from build123d import *

# Parameters (mm, degrees)
F0_W         = 76.2
F0_H         = 101.6
F1_DEPTH     = 38.1
F2_W         = 69.85
F2_H         = 95.25
F3_DEPTH     = 34.925
F4_W         = 72.39
F4_H         = 97.79
F4_W_2       = 69.85
F4_H_2       = 95.25
F5_DEPTH     = 3.175
F6_W         = 76.2
F6_H         = 101.6
F6_W_2       = 73.66
F6_H_2       = 99.06
F7_DEPTH     = 3.175
F8_T1_DEPTH  = 110.49
F8_T3_DEPTH  = 85.09
F8_T5_DEPTH  = 99.06
F8_T7_DEPTH  = 73.66
F8_T13_DEPTH = 105.41
F8_T19_DEPTH = 80.01
F8_T28_DEPTH = 105.41
F8_T34_DEPTH = 80.01
F8_T43_DEPTH = 80.01
F8_T49_DEPTH = 105.41
F8_T58_DEPTH = 105.41
F8_T64_DEPTH = 80.01


# Not quite as in the source:
# - a fillet or chamfer that OpenCascade refuses, or shapes differently, is made with other operations: its cross-section is extruded or revolved along the edge and cut away or added


with BuildPart() as f1:
    # F0 (on Top) → F1 (new body)
    with BuildSketch(Plane.XY):
        Rectangle(F0_W, F0_H)
    extrude(amount=F1_DEPTH)

    # F2 (on face) → F3 (cut)
    with BuildSketch(Plane.XY.offset(38.1)):
        Rectangle(F2_W, F2_H)
    extrude(amount=-F3_DEPTH, mode=Mode.SUBTRACT)

    # F4 (on face) → F5 (join)
    with BuildSketch(Plane.XY.offset(38.1)):
        Rectangle(F4_W, F4_H)
        Rectangle(F4_W_2, F4_H_2, mode=Mode.SUBTRACT)
    extrude(amount=F5_DEPTH)

    # F6 (on face) → F7 (join)
    with BuildSketch(Plane(origin=(0, 0, 0), x_dir=(1, 0, 0), z_dir=(0, 0, -1))):
        Rectangle(F6_W, F6_H)
        Rectangle(F6_W_2, F6_H_2, mode=Mode.SUBTRACT)
    extrude(amount=F7_DEPTH)

    # F8: fillet of radius 2.54 on 8 edges, made by hand

    # F8_s2 → F8_t1 (cut)
    with BuildSketch(Plane.XZ.offset(-55.245)):
        with BuildLine():
            ThreePointArc((-33.655, 41.275), (-35.4510512242, 40.5310512242), (-36.195, 38.735))
            Line((-36.195, 38.735), (-36.195, 41.275))
            Line((-36.195, 41.275), (-33.655, 41.275))
        make_face()
        with BuildLine():
            ThreePointArc((36.195, 38.735), (35.4510512242, 40.5310512242), (33.655, 41.275))
            Line((33.655, 41.275), (36.195, 41.275))
            Line((36.195, 41.275), (36.195, 38.735))
        make_face()
    extrude(amount=F8_T1_DEPTH, mode=Mode.SUBTRACT)

    # F8_s4 → F8_t3 (cut)
    with BuildSketch(Plane.YZ.offset(-42.545)):
        with BuildLine():
            ThreePointArc((-46.355, 41.275), (-48.1510512242, 40.5310512242), (-48.895, 38.735))
            Line((-48.895, 38.735), (-48.895, 41.275))
            Line((-48.895, 41.275), (-46.355, 41.275))
        make_face()
        with BuildLine():
            ThreePointArc((46.355, 41.275), (48.1510512242, 40.5310512242), (48.895, 38.735))
            Line((48.895, 38.735), (48.895, 41.275))
            Line((48.895, 41.275), (46.355, 41.275))
        make_face()
    extrude(amount=F8_T3_DEPTH, mode=Mode.SUBTRACT)

    # F8_s6 → F8_t5 (cut)
    with BuildSketch(Plane.XZ.offset(-49.53)):
        with BuildLine():
            ThreePointArc((-39.37, -3.175), (-37.5739487758, -2.4310512242), (-36.83, -0.635))
            Line((-36.83, -0.635), (-36.83, -3.175))
            Line((-36.83, -3.175), (-39.37, -3.175))
        make_face()
        with BuildLine():
            ThreePointArc((39.37, -3.175), (37.5739487758, -2.4310512242), (36.83, -0.635))
            Line((36.83, -0.635), (36.83, -3.175))
            Line((36.83, -3.175), (39.37, -3.175))
        make_face()
    extrude(amount=F8_T5_DEPTH, mode=Mode.SUBTRACT)

    # F8_s8 → F8_t7 (cut)
    with BuildSketch(Plane.YZ.offset(-36.83)):
        with BuildLine():
            ThreePointArc((-52.07, -3.175), (-50.2739487758, -2.4310512242), (-49.53, -0.635))
            Line((-49.53, -0.635), (-49.53, -3.175))
            Line((-49.53, -3.175), (-52.07, -3.175))
        make_face()
        with BuildLine():
            ThreePointArc((52.07, -3.175), (50.2739487758, -2.4310512242), (49.53, -0.635))
            Line((49.53, -0.635), (49.53, -3.175))
            Line((49.53, -3.175), (52.07, -3.175))
        make_face()
    extrude(amount=F8_T7_DEPTH, mode=Mode.SUBTRACT)


with BuildPart() as f8_tool11:
    # F8_s12 → F8_t13 (new body)
    with BuildSketch(Plane.XZ.offset(-55.88)):
        with BuildLine():
            ThreePointArc((-39.37, -3.175), (-37.5739487758, -2.4310512242), (-36.83, -0.635))
            Line((-36.83, -0.635), (-36.83, -3.175))
            Line((-36.83, -3.175), (-39.37, -3.175))
        make_face()
    extrude(amount=F8_T13_DEPTH)

    split(bisect_by=Plane.XZ.offset(-49.53), keep=Keep.BOTTOM)

    split(bisect_by=Plane.YZ.offset(-38.1), keep=Keep.TOP)

    split(bisect_by=Plane.XZ.offset(-50.8), keep=Keep.TOP)


with BuildPart() as f8_tool17:
    # F8_s18 → F8_t19 (new body)
    with BuildSketch(Plane.YZ.offset(36.83)):
        with BuildLine():
            ThreePointArc((52.07, -3.175), (50.2739487758, -2.4310512242), (49.53, -0.635))
            Line((49.53, -0.635), (49.53, -3.175))
            Line((49.53, -3.175), (52.07, -3.175))
        make_face()
    extrude(amount=-F8_T19_DEPTH)

    split(bisect_by=Plane.YZ.offset(-36.83), keep=Keep.BOTTOM)

    split(bisect_by=Plane.YZ.offset(-38.1), keep=Keep.TOP)

    split(bisect_by=Plane.XZ.offset(-50.8), keep=Keep.TOP)


with BuildPart() as f8_tool11_1:
    add(f8_tool11.part)

    # F8_t23: intersect F8_tool17
    add(f8_tool17.part, mode=Mode.INTERSECT)


with BuildPart() as f1_1:
    add(f1.part)

    # F8_t9: cut F8_tool11
    add(f8_tool11_1.part, mode=Mode.SUBTRACT)


with BuildPart() as f8_tool26:
    # F8_s27 → F8_t28 (new body)
    with BuildSketch(Plane.XZ.offset(-49.53)):
        with BuildLine():
            ThreePointArc((-39.37, -3.175), (-37.5739487758, -2.4310512242), (-36.83, -0.635))
            Line((-36.83, -0.635), (-36.83, -3.175))
            Line((-36.83, -3.175), (-39.37, -3.175))
        make_face()
    extrude(amount=F8_T28_DEPTH)

    split(bisect_by=Plane.XZ.offset(49.53), keep=Keep.TOP)

    split(bisect_by=Plane.YZ.offset(-38.1), keep=Keep.TOP)

    split(bisect_by=Plane.XZ.offset(50.8), keep=Keep.BOTTOM)


with BuildPart() as f8_tool32:
    # F8_s33 → F8_t34 (new body)
    with BuildSketch(Plane.YZ.offset(-43.18)):
        with BuildLine():
            ThreePointArc((-52.07, -3.175), (-50.2739487758, -2.4310512242), (-49.53, -0.635))
            Line((-49.53, -0.635), (-49.53, -3.175))
            Line((-49.53, -3.175), (-52.07, -3.175))
        make_face()
    extrude(amount=F8_T34_DEPTH)

    split(bisect_by=Plane.YZ.offset(-36.83), keep=Keep.BOTTOM)

    split(bisect_by=Plane.YZ.offset(-38.1), keep=Keep.TOP)

    split(bisect_by=Plane.XZ.offset(50.8), keep=Keep.BOTTOM)


with BuildPart() as f8_tool26_1:
    add(f8_tool26.part)

    # F8_t38: intersect F8_tool32
    add(f8_tool32.part, mode=Mode.INTERSECT)


with BuildPart() as f1_2:
    add(f1_1.part)

    # F8_t24: cut F8_tool26
    add(f8_tool26_1.part, mode=Mode.SUBTRACT)


with BuildPart() as f8_tool41:
    # F8_s42 → F8_t43 (new body)
    with BuildSketch(Plane.YZ.offset(-36.83)):
        with BuildLine():
            ThreePointArc((-52.07, -3.175), (-50.2739487758, -2.4310512242), (-49.53, -0.635))
            Line((-49.53, -0.635), (-49.53, -3.175))
            Line((-49.53, -3.175), (-52.07, -3.175))
        make_face()
    extrude(amount=F8_T43_DEPTH)

    split(bisect_by=Plane.YZ.offset(38.1), keep=Keep.BOTTOM)

    split(bisect_by=Plane.YZ.offset(36.83), keep=Keep.TOP)

    split(bisect_by=Plane.XZ.offset(50.8), keep=Keep.BOTTOM)


with BuildPart() as f8_tool47:
    # F8_s48 → F8_t49 (new body)
    with BuildSketch(Plane.XZ.offset(55.88)):
        with BuildLine():
            ThreePointArc((39.37, -3.175), (37.5739487758, -2.4310512242), (36.83, -0.635))
            Line((36.83, -0.635), (36.83, -3.175))
            Line((36.83, -3.175), (39.37, -3.175))
        make_face()
    extrude(amount=-F8_T49_DEPTH)

    split(bisect_by=Plane.YZ.offset(38.1), keep=Keep.BOTTOM)

    split(bisect_by=Plane.XZ.offset(49.53), keep=Keep.TOP)

    split(bisect_by=Plane.XZ.offset(50.8), keep=Keep.BOTTOM)


with BuildPart() as f8_tool41_1:
    add(f8_tool41.part)

    # F8_t53: intersect F8_tool47
    add(f8_tool47.part, mode=Mode.INTERSECT)


with BuildPart() as f1_3:
    add(f1_2.part)

    # F8_t39: cut F8_tool41
    add(f8_tool41_1.part, mode=Mode.SUBTRACT)


with BuildPart() as f8_tool56:
    # F8_s57 → F8_t58 (new body)
    with BuildSketch(Plane.XZ.offset(49.53)):
        with BuildLine():
            ThreePointArc((39.37, -3.175), (37.5739487758, -2.4310512242), (36.83, -0.635))
            Line((36.83, -0.635), (36.83, -3.175))
            Line((36.83, -3.175), (39.37, -3.175))
        make_face()
    extrude(amount=-F8_T58_DEPTH)

    split(bisect_by=Plane.YZ.offset(38.1), keep=Keep.BOTTOM)

    split(bisect_by=Plane.XZ.offset(-49.53), keep=Keep.BOTTOM)

    split(bisect_by=Plane.XZ.offset(-50.8), keep=Keep.TOP)


with BuildPart() as f8_tool62:
    # F8_s63 → F8_t64 (new body)
    with BuildSketch(Plane.YZ.offset(43.18)):
        with BuildLine():
            ThreePointArc((52.07, -3.175), (50.2739487758, -2.4310512242), (49.53, -0.635))
            Line((49.53, -0.635), (49.53, -3.175))
            Line((49.53, -3.175), (52.07, -3.175))
        make_face()
    extrude(amount=-F8_T64_DEPTH)

    split(bisect_by=Plane.YZ.offset(38.1), keep=Keep.BOTTOM)

    split(bisect_by=Plane.YZ.offset(36.83), keep=Keep.TOP)

    split(bisect_by=Plane.XZ.offset(-50.8), keep=Keep.TOP)


with BuildPart() as f8_tool56_1:
    add(f8_tool56.part)

    # F8_t68: intersect F8_tool62
    add(f8_tool62.part, mode=Mode.INTERSECT)


with BuildPart() as f1_4:
    add(f1_3.part)

    # F8_t54: cut F8_tool56
    add(f8_tool56_1.part, mode=Mode.SUBTRACT)


solid = f1_4.part
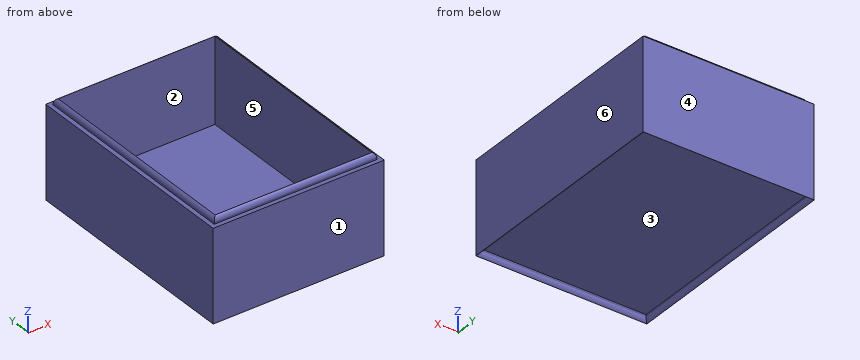
Read the model definition and answer for the solid it produces. Units are mm, in the model's axes. Face numbers are marked on the shaded views. A direction names the side the tool comes from. Give positions to 0.01 mm unless a question says otherwise; leave off trailing zeros. Write each loop counter-clockwise with the first axis right and the second up, starting at its lowest first coordinate (ties: lowest second). Pieces come first, ordered by that corner, then holes. Notation, with made-up numbers: (21, -23) - (73, -23) arc R15 cw to (73, 3) - close; hole circle Ø5 at (-35.5, 89.25). An arc over 180 degrees is marked (long way). Use CSV: the item, a comma, the result in double quotes. Start each with the question number.
Item 1: Flat-ended cylindrical pins translate along their axes: P1, Ø4, axis at x = 3.5, y = 20, coming from the -Z side; P2, Ø21, axis at x = 1.5, y = 12, coming from the +Z side (3 decimals); P3, Ø0.5, axis at y = -17, z = 38.5, coming from the +X side (3 decimals). Find the tip coordinate at first contact, or state that the pin passes through.
Item 2: The part is cut by section A-A, the plane y = 1. Give the vertices of the cut face in (x, z) (3 decimals).
Item 3: The part is cut by section B-B, the plane x = 9. Give the vertices of the cut face in (y, z) (3 decimals).
Item 4: The mould has two halves that part along X. Classify the marked faces 4, 5 and 6: pulls with the +X half, pulls with the -X half, needs draft (parallel to the pull), parting line crosses it, or undercut.
Item 5: Consider line 1 (X direction, y = -46, z = 16.5) (3 decimals); line 2 (Y direction, x = 16, z = 11) (3 decimals); line 3 (Z direction, x = -0.5, y = 4) (3 decimals). Determine where each line is inside the solid, lowest interval first.
Item 6: The part is cut by section C-C, the plane z = 17. Give the vertices of the cut face in (x, y) (3 decimals).
Item 7: For the marked faces 1, 2 and 3, determine the directions among +Z, -Z, +X, -X, +Y, -Y from which every point of the face is accessible in a straight line to the end or side of a thin tool.
Taken from the geometry:
1,P1,"z = 0"
1,P2,"z = 3.175"
1,P3,"x = 36.195"
2,outline,"(-38.1, -2.835) arc R2.54 ccw to (-36.83, -0.635) - (-36.83, 0) - (36.83, 0) - (36.83, -0.635) arc R2.54 ccw to (38.1, -2.835) - (38.1, 38.1) - (36.195, 38.1) - (36.195, 38.735) arc R2.54 ccw to (34.925, 40.935) - (34.925, 3.175) - (-34.925, 3.175) - (-34.925, 40.935) arc R2.54 ccw to (-36.195, 38.735) - (-36.195, 38.1) - (-38.1, 38.1) - close"
3,outline,"(-50.8, -2.835) arc R2.54 ccw to (-49.53, -0.635) - (-49.53, 0) - (49.53, 0) - (49.53, -0.635) arc R2.54 ccw to (50.8, -2.835) - (50.8, 38.1) - (48.895, 38.1) - (48.895, 38.735) arc R2.54 ccw to (47.625, 40.935) - (47.625, 3.175) - (-47.625, 3.175) - (-47.625, 40.935) arc R2.54 ccw to (-48.895, 38.735) - (-48.895, 38.1) - (-50.8, 38.1) - close"
4,face 4,"needs draft"
4,face 5,"undercut"
4,face 6,"pulls with the +X half"
5,line 1,"-38.1 to -34.925, 34.925 to 38.1"
5,line 2,"-50.8 to -47.625, 47.625 to 50.8"
5,line 3,"0 to 3.175"
6,outline,"(-38.1, -50.8) - (38.1, -50.8) - (38.1, 50.8) - (-38.1, 50.8) - close; hole (-34.925, -47.625) - (34.925, -47.625) - (34.925, 47.625) - (-34.925, 47.625) - close"
7,face 1,"+Z, -Z, +X, -X, -Y"
7,face 2,"+Z"
7,face 3,"-Z"
